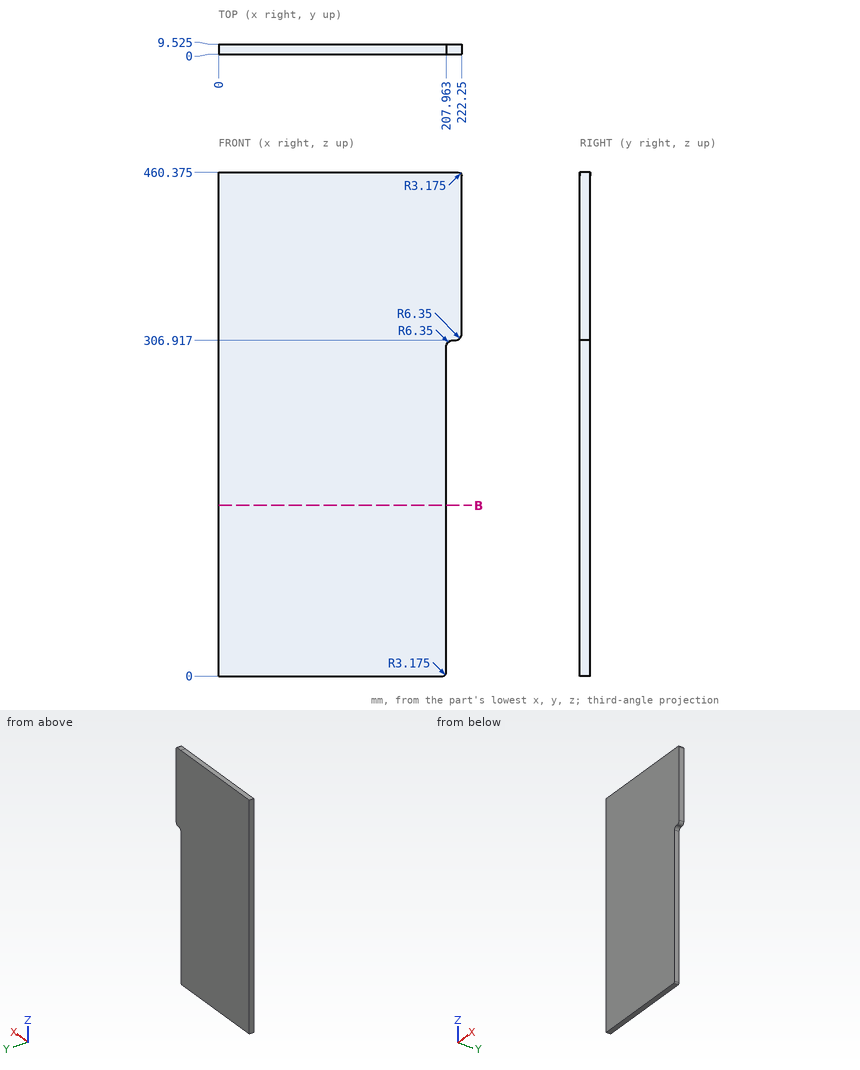
Can you work these out from the drawing? Everything is in mm from the part's minimum corner. Round coordinates to 2 decimals unless told otherwise and drop trailing zeros. Write each loop counter-clockwise with the first axis right and the second up, starting at its lowest first coordinate (ties: lowest second). Pieces come first, ordered by that corner, then holes. Notation, with made-up numbers: (16.25, -29.5) - (41.25, -29.5) arc R27 ccw to (41.25, 1.5) - close; hole circle Ø8 at (25.25, 67). An arc over 180 degrees is marked (long way). Write each question's results on one line, items separated by ' | '. Start each with the question number.
1) Please list where these lines run through material, in increasing order: line 1 (X direction, y = 8.5, z = 259); line 2 (X direction, y = 3.25, z = 304.5) (1 decimal).
2) For pin 1 Ø5 at (y, z) = (4, 187) entering from +X; pin 2 Ø1.7 at (x, y) = (215, 7) entering from -Z (1 decimal), each with a flat end and sliding along its axis, tell me the tip position at first contact or that it passes through.
3) Suppose I cut it at B-B (z = 156). List the corners of the cut face in (x, y) for me (1 decimal).
Here are the results:
1) line 1: x = 0 to 207.96 | line 2: x = 0 to 209.3
2) pin 1: stops at x = 207.96 | pin 2: stops at z = 306.9
3) outline: (0, 0) - (208, 0) - (208, 9.5) - (0, 9.5) - close
